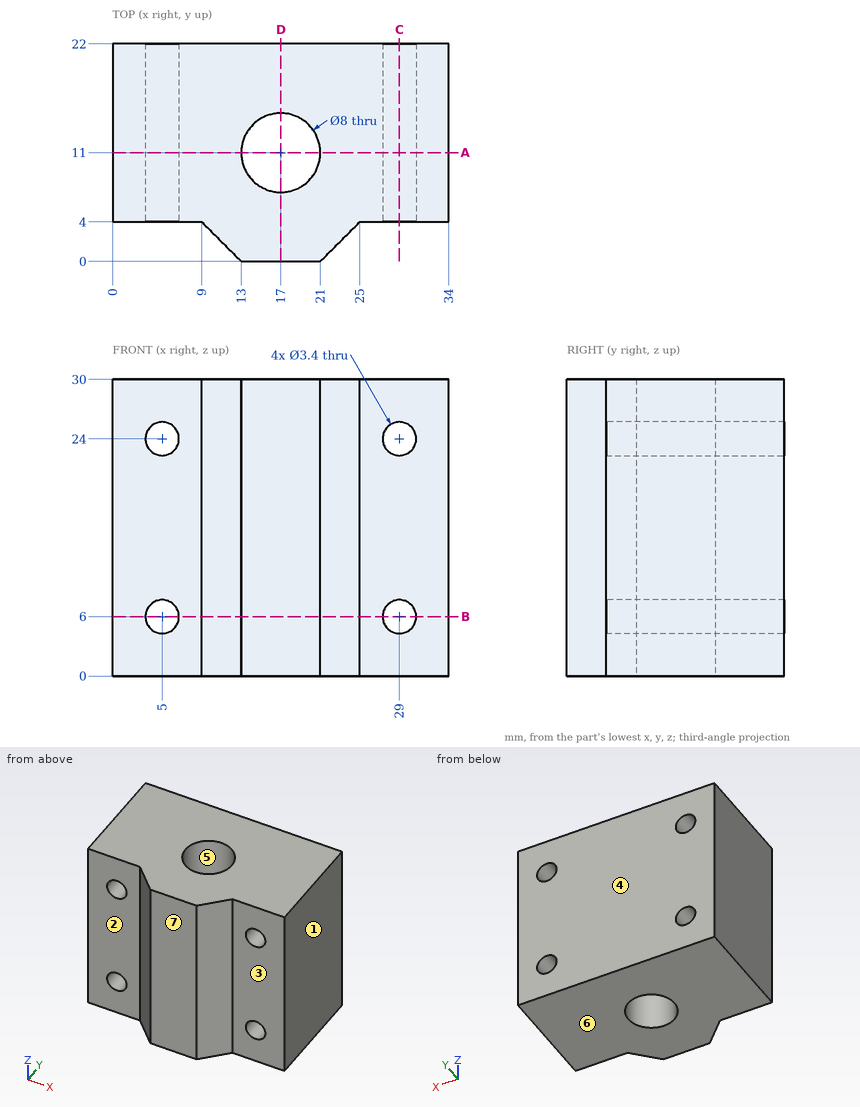
The drawing under review shows one solid part. Ordinate dimensions are in mm from its lowest x, y, z. A direction names the side the tool comes from. Round coordinates to 2 decimals unless told otherwise and drop trailing zeros. Loops run counter-clockwise (first coordinate to the right, second up) from the corner with the lowest first, then second, coordinate; pieces in that order, holes last. Notation, with made-up numbers: (57.25, 72.25) - (74.25, 72.25) arc R15 cw to (74.25, 83.25) - close; hole circle Ø7 at (-14.75, 5). An arc over 180 degrees is marked (long way). Use a Markdown table: item, result. Add a question column.
Q1. Add section D-D (x = 17). State the section outline as (y, z) points.
Q2. The part is to be moulded in two halves that separate along Y. For the marked faces 4, 5, 6 and 7, say which applies: pulls with the +Y half, pulls with the -Y half, needs draft (parallel to the pull), parting line crosses it, or undercut.
Q3. Add section A-A (y = 11). State the section outline as (x, z) points.
Q4. Insertion check: pin 1 Ø2.5 at (x, z) = (6.5, 21.5) entering from -Y. The pin has a flat end and moves straight along its axis. Give the tip position at first contact, or say it passes through.
Q5. For probe 1 along X at (y, z) = (16, 6); probe 2 along Y at (x, z) = (17, 16.25); probe 3 along X at (y, z) = (12, 6.75), list the stretches that pass through material, from the lowest coordinate up.
Q6. Machinability: for the marked faces 1, 2 and 3, which of the approach directions +Z, -Z, +X, -X, +Y, -Y give a long, thin tool a straight path to every point of the face, cutting with its end or side? Answer none if there is none.
Q7. Add section B-B (z = 6). State the section outline as (x, y) points.
Q8. Add section C-C (x = 29). State the section outline as (y, z) points.
Worked answers:
| question | item | result |
|---|---|---|
| 1 | outline | (0, 0) - (7, 0) - (7, 30) - (0, 30) - close; (15, 0) - (22, 0) - (22, 30) - (15, 30) - close |
| 2 | face 4 | pulls with the +Y half |
| 2 | face 5 | undercut |
| 2 | face 6 | needs draft |
| 2 | face 7 | pulls with the -Y half |
| 3 | outline | (0, 0) - (13, 0) - (13, 30) - (0, 30) - close; (21, 0) - (34, 0) - (34, 30) - (21, 30) - close; hole circle Ø3.4 at (5, 6); hole circle Ø3.4 at (5, 24); hole circle Ø3.4 at (29, 6); hole circle Ø3.4 at (29, 24) |
| 4 | pin 1 | y = 4 |
| 5 | probe 1 | 0 to 3.3, 6.7 to 27.3, 30.7 to 34 |
| 5 | probe 2 | 0 to 7, 15 to 22 |
| 5 | probe 3 | 0 to 3.47, 6.53 to 13.13, 20.87 to 27.47, 30.53 to 34 |
| 6 | face 1 | +Z, -Z, +X, +Y, -Y |
| 6 | face 2 | +Z, -Z, -X, -Y |
| 6 | face 3 | +Z, -Z, +X, -Y |
| 7 | outline | (0, 4) - (3.3, 4) - (3.3, 22) - (0, 22) - close; (6.7, 4) - (9, 4) - (13, 0) - (21, 0) - (25, 4) - (27.3, 4) - (27.3, 22) - (6.7, 22) - close; (30.7, 4) - (34, 4) - (34, 22) - (30.7, 22) - close; hole circle Ø8 at (17, 11) |
| 8 | outline | (4, 0) - (22, 0) - (22, 4.3) - (4, 4.3) - close; (4, 7.7) - (22, 7.7) - (22, 22.3) - (4, 22.3) - close; (4, 25.7) - (22, 25.7) - (22, 30) - (4, 30) - close |
